Here's the drawing with two shaded views (mm, measured from the low corner). I have some questions. Coordinates: 2 decimals unless noted, no trailing zeros. Loops run counter-clockwise (first coordinate to the right, second up) from the corner with the lowest first, then second, coordinate; pieces in that order, holes last. Notation, with made-up numbers: (49, -29) -> (75, -29) arc R23 ccw to (75, 2) -> close; hole circle Ø10 at (48, -16.75). An arc over 180 degrees is marked (long way). Answer as a JSON object with one key per item and string values. Group by question number.
1) I'm going to push flat-ended pins straight in: pin 1 (5 mm diameter, centred on x = 18.5, z = 35.5, fed in from +Y); pin 2 (2 mm diameter, centred on y = 22.5, z = 17, fed in from +X). Where does each tip first touch, or does it pass through?
2) If we mould it in two halves opening along Z, with no side actions, what happens to the marked faces 1, 2, 3 and 4? For each: +Z half, -Z half, draft (parallel to the pull), parting line (faces both ways), or undercut.
3) I want a section at C-C (z = 13). Write out the boundary of the cut face in (x, y), then the cut area to 3 significant figures.
4) I need wall thicknesses on probe 1 along Z at (x, y) = (48, 25); probe 2 along X at (y, z) = (21.5, 27.5); probe 3 along X at (y, z) = (48, 23.5). Which ranges of each line are inside material? Lowest first, please. Write a range as [from, to].
5) I want a section at A-A (y = 25). Write out the boundary of the cut face in (x, z), then the cut area to 3 significant figures.
6) I want a section at B-B (x = 47.5). Write out the boundary of the cut face in (y, z).
7) I want a section at D-D (x = 41.5). Write out the boundary of the cut face in (y, z), then the cut area to 3 significant figures.
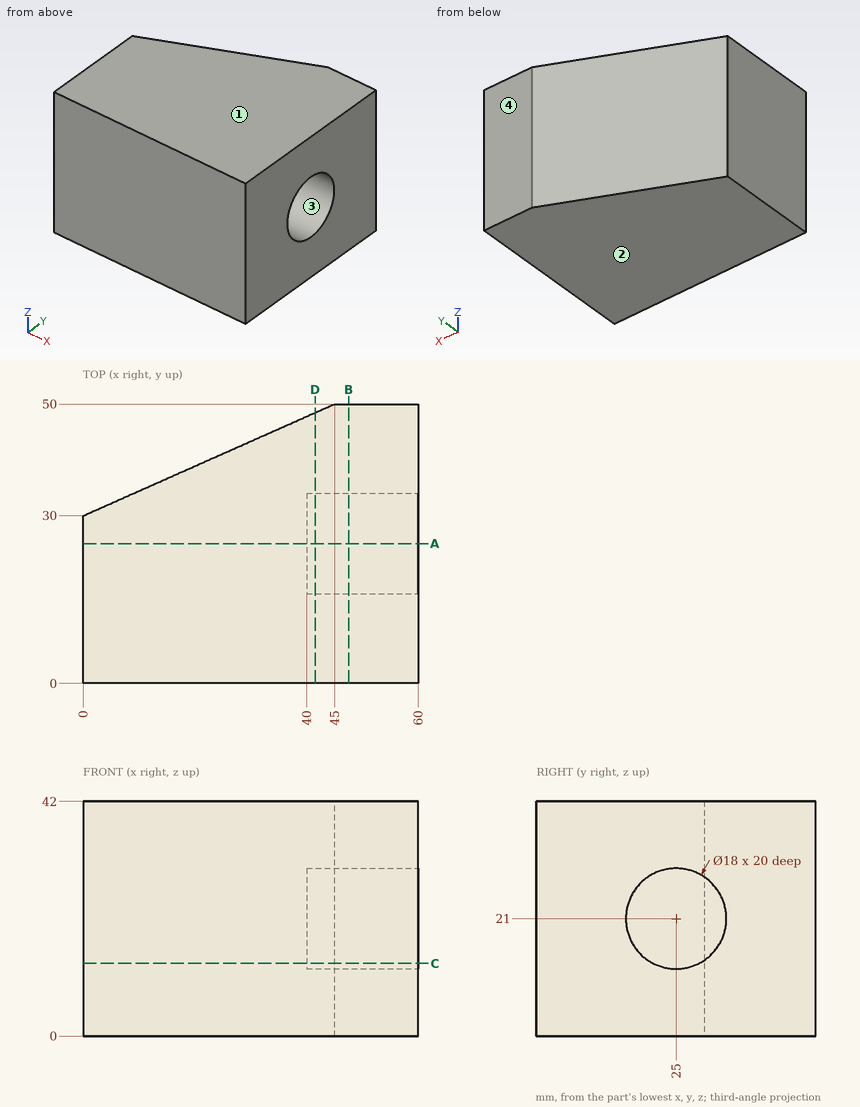
Determined:
{
 "1": {"pin 1": "y = 39.33", "pin 2": "x = 40"},
 "2": {"face 1": "+Z half", "face 2": "-Z half", "face 3": "undercut", "face 4": "draft"},
 "3": {"outline": "(0, 0) -> (60, 0) -> (60, 20.88) -> (40, 20.88) -> (40, 29.12) -> (60, 29.12) -> (60, 50) -> (45, 50) -> (0, 30) -> close", "area": "2,390 mm^2"},
 "4": {"probe 1": "[0, 12], [30, 42]", "probe 2": "[0, 40]", "probe 3": "[40.5, 60]"},
 "5": {"outline": "(0, 0) -> (60, 0) -> (60, 12) -> (40, 12) -> (40, 30) -> (60, 30) -> (60, 42) -> (0, 42) -> close", "area": "2,160 mm^2"},
 "6": {"outline": "(0, 0) -> (50, 0) -> (50, 42) -> (0, 42) -> close; hole circle Ø18 at (25, 21)"},
 "7": {"outline": "(0, 0) -> (48.44, 0) -> (48.44, 42) -> (0, 42) -> close; hole circle Ø18 at (25, 21)", "area": "1,780 mm^2"}
}
